Geometry: final body of the model. Coordinates: model frame, mm. A direction names the side the tool comes from. Coordinates: 2 decimals unless noted, no trailing zeros. Order: outer loops, then holes, each group sorted by start corner. A loop starts at its lowest first (then second) coordinate and runs counter-clockwise, first axis right, second up. Notation, with made-up numbers: M 13.25,-11 L 64.25,-11 A22 cw 64.25,4 Z; hole C 66,-21 d4. An arc over 180 degrees is marked long. Use CSV: the item, a comma, the result in double quotes. Start each with the question number.
Q1. Access query for faces 4 (the face through (37, 0, 9)), 5 (the face through (-1, 12.35, 9)). Directions: +Z, -Z, +X, -X, +Y, -Y. A direction counts if a zero-diameter tool reaches every point of the face in a straight line with its end or side. Return the directions, or none.
Q2. Section query A-A, the plane z = 12. Output: boundary loops of the cut face in (x, y), and give its area (3 significant figures).
Q3. Section query C-C, the plane y = 6.75. Output: boundary loops of the cut face in (x, z).
Q4. Section query B-B, the plane x = -30.5. Output: boundary loops of the cut face in (y, z).
Q5. Mould query, pull axis X, two halves, no side actions, for faces 1 (the face through (-38.6, 0, 9)), 2 (the face through (-1, -10.75, 9)), 3 (the face through (-6, -11, 19)). Classes: +X half, -X half, draft (parallel to the pull), parting line (faces both ways), or undercut.
Q6. Ray query, probe 1 along Y at (x, z) = (-6, 16.25); probe 2 along X at (y, z) = (10.5, 13); probe 3 along Z at (x, y) = (9, -7.75). Return the intervals inside material, ascending.
Q7. First-contact query: P1, Ø6, axis at x = 5, y = 0, coming from the +Z side. Flat tip, straight axial feed; report the tip coordinate or a pass-through.
from build123d import *

# Parameters (mm, degrees)
SKETCH1_W           = 77.2
SKETCH1_H           = 24.7
SKETCH1_W_2         = 74
SKETCH1_H_2         = 21.5
BOSS_EXTRUDE1_DEPTH = 19
SKETCH1_2_W         = 77.2
SKETCH1_2_H         = 24.7
SKETCH1_2_W_2       = 74
SKETCH1_2_H_2       = 21.5
BOSS_EXTRUDE2_DEPTH = 1.2


with BuildPart() as part:
    # Sketch1 → Boss-Extrude1 (new body)
    with BuildSketch(Plane.XY):
        Rectangle(SKETCH1_W, SKETCH1_H)
        Rectangle(SKETCH1_W_2, SKETCH1_H_2, mode=Mode.SUBTRACT)
    extrude(amount=BOSS_EXTRUDE1_DEPTH)

    # Sketch1_2 → Boss-Extrude2 (add)
    # profile 1 of 2: a face of its own
    with BuildSketch(Plane.XY):
        Rectangle(SKETCH1_2_W, SKETCH1_2_H)
        Rectangle(SKETCH1_2_W_2, SKETCH1_2_H_2, mode=Mode.SUBTRACT)
    # profile 2 of 2: a face of its own
    with BuildSketch(Plane.XY):
        Rectangle(SKETCH1_2_W_2, SKETCH1_2_H_2)
    extrude(amount=-BOSS_EXTRUDE2_DEPTH)


solid = part.part
Responses:
1,face 4,"+Z"
1,face 5,"+Z, -Z, +X, -X, +Y"
2,outline,"M -38.6,-12.35 L 38.6,-12.35 L 38.6,12.35 L -38.6,12.35 Z; hole M -37,-10.75 L 37,-10.75 L 37,10.75 L -37,10.75 Z"
2,area,"316 mm²"
3,outline,"M -38.6,-1.2 L 38.6,-1.2 L 38.6,19 L 37,19 L 37,0 L -37,0 L -37,19 L -38.6,19 Z"
4,outline,"M -12.35,-1.2 L 12.35,-1.2 L 12.35,19 L 10.75,19 L 10.75,0 L -10.75,0 L -10.75,19 L -12.35,19 Z"
5,face 1,"-X half"
5,face 2,"undercut"
5,face 3,"draft"
6,probe 1,"y = -12.35 to -10.75, 10.75 to 12.35"
6,probe 2,"x = -38.6 to -37, 37 to 38.6"
6,probe 3,"z = -1.2 to 0"
7,P1,"stops at z = 0"
